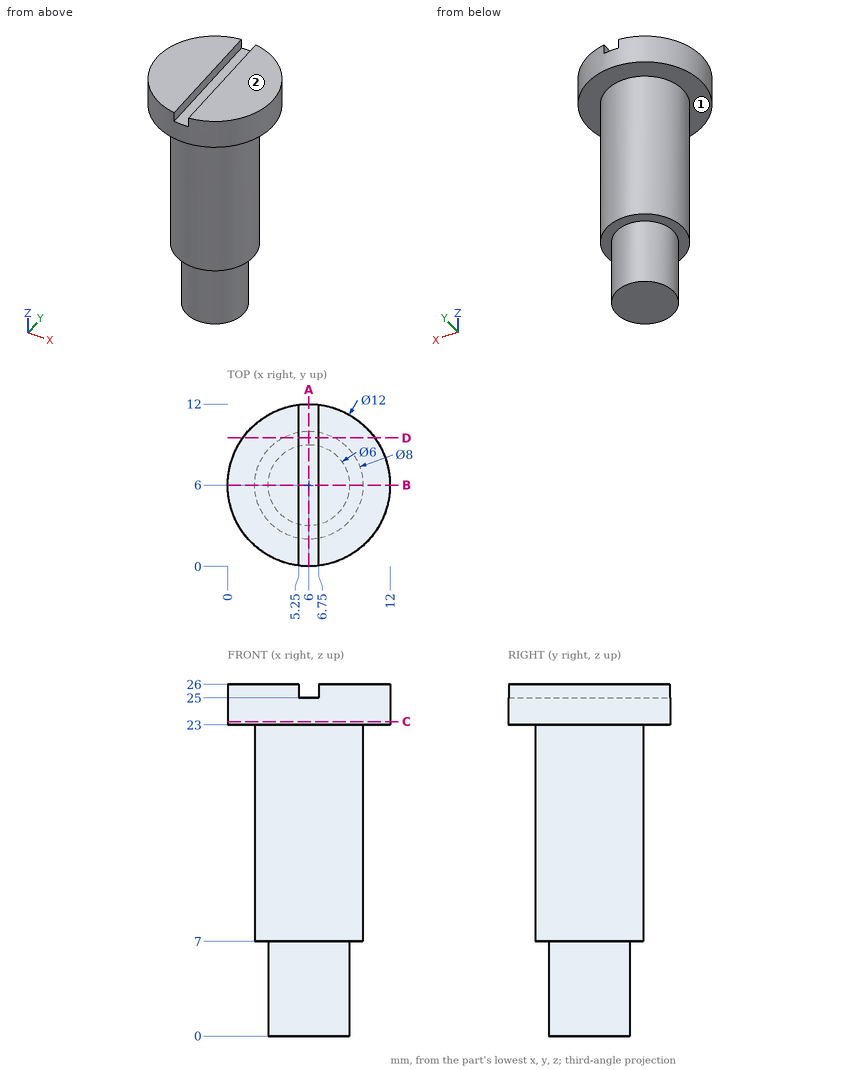
Can you work these out from the drawing? Everything is in mm from the part's minimum corner. A direction names the side the tool comes from. Coordinates: 2 decimals unless noted, no trailing zeros. Loops run counter-clockwise (first coordinate to the right, second up) from the corner with the lowest first, then second, coordinate; pieces in that order, holes last.
1. For P1, Ø1, axis at x = 7, z = 4, coming from the -Y side; P2, Ø0.5, axis at y = 3, z = 25.5, coming from the +X side; P3, Ø1, axis at y = 7.5, z = 20, coming from the +X side, each with a flat end and sliding along its axis, tell me the tip position at first contact or that it passes through.
2. Imagine slicing it at C-C, the plane z = 23.25. Please give me the cut outline in (x, y), and give its area (3 significant figures).
3. I need wall thicknesses on L1, parallel to Z at x = 4, y = 9.25; L2, parallel to Z at x = 6, y = 4.25; L3, parallel to X at y = 4.25, z = 10.5. Which ranges of each line are inside material? Lowest first, please.
4. Imagine slicing it at B-B, the plane y = 6. Please give me the cut outline in (x, z), and give its area (4 significant figures).
5. Imagine slicing it at A-A, the plane x = 6. Please give me the cut outline in (y, z).
6. For the marked faces 1 and 2, which set-ups out of +Z, -Z, +X, -X, +Y, -Y let a thin tool reach every point of the face, with its end or its side?
7. Imagine slicing it at D-D, the plane y = 9.5. Please give me the cut outline in (x, z), and give its area (3 significant figures).
Taken from the geometry:
1. P1: stops at y = 3.04
1. P2: stops at x = 11.33
1. P3: stops at x = 9.87
2. outline: circle Ø12 at (6, 6)
2. area: 113 mm2
3. L1: z = 7 to 26
3. L2: z = 0 to 25
3. L3: x = 2.4 to 9.6
4. outline: (0, 23) - (2, 23) - (2, 7) - (3, 7) - (3, 0) - (9, 0) - (9, 7) - (10, 7) - (10, 23) - (12, 23) - (12, 26) - (6.75, 26) - (6.75, 25) - (5.25, 25) - (5.25, 26) - (0, 26) - close
4. area: 204.5 mm2
5. outline: (0, 23) - (2, 23) - (2, 7) - (3, 7) - (3, 0) - (9, 0) - (9, 7) - (10, 7) - (10, 23) - (12, 23) - (12, 25) - (0, 25) - close
6. face 1: -Z
6. face 2: +Z, +X, -X, +Y, -Y
7. outline: (1.13, 23) - (4.06, 23) - (4.06, 7) - (7.94, 7) - (7.94, 23) - (10.87, 23) - (10.87, 26) - (6.75, 26) - (6.75, 25) - (5.25, 25) - (5.25, 26) - (1.13, 26) - close
7. area: 89.7 mm2
